from build123d import *

# Parameters (mm, degrees)
ESQUISSE1_W             = 120
ESQUISSE1_H             = 90
BOSS_EXTRU_1_DEPTH      = 2
ESQUISSE2_W             = 115
ESQUISSE2_H             = 85
ESQUISSE2_W_2           = 111
ESQUISSE2_H_2           = 82.04347826
BOSS_EXTRU_2_DEPTH      = 2
ENL_V_MAT_EXTRU_1_DEPTH = 2
CONG_1_R                = 3
CONG_2_R                = 0.5


with BuildPart() as part:
    # Esquisse1 → Boss.-Extru.1 (new body)
    with BuildSketch(Plane.XY):
        Rectangle(ESQUISSE1_W, ESQUISSE1_H)
    extrude(amount=BOSS_EXTRU_1_DEPTH)

    # Esquisse2 → Boss.-Extru.2 (add)
    with BuildSketch(Plane.XY.offset(2)):
        Rectangle(ESQUISSE2_W, ESQUISSE2_H)
        Rectangle(ESQUISSE2_W_2, ESQUISSE2_H_2, mode=Mode.SUBTRACT)
    extrude(amount=BOSS_EXTRU_2_DEPTH)

    # Esquisse3 → Enlèv. mat.-Extru.1 (cut)
    with BuildSketch(Plane(origin=(0, 0, 0), x_dir=(-1, 0, 0), z_dir=(0, 0, -1))):
        with BuildLine():
            Line((5.548380707, 39.874958244), (25.548380707, 39.874958244))
            ThreePointArc((25.548380707, 39.874958244), (30.548380707, 34.874958244), (25.548380707, 29.874958244))
            Line((25.548380707, 29.874958244), (5.548380707, 29.874958244))
            ThreePointArc((5.548380707, 29.874958244), (0.548380707, 34.874958244), (5.548380707, 39.874958244))
        make_face()
    extrude(amount=-ENL_V_MAT_EXTRU_1_DEPTH, mode=Mode.SUBTRACT)

    # Congé1
    cong_1_edges = [part.edges().sort_by_distance(p)[0] for p in [
        (-60, 45, 1),
        (60, 45, 1),
        (60, -45, 1),
        (-60, -45, 1),
    ]]
    fillet(cong_1_edges, radius=CONG_1_R)

    # Congé2
    cong_2_edges = [part.edges().sort_by_distance(p)[0] for p in [
        (-57.5, 42.5, 3),
        (-57.5, -42.5, 3),
        (57.5, -42.5, 3),
        (57.5, 42.5, 3),
    ]]
    fillet(cong_2_edges, radius=CONG_2_R)


solid = part.part
Work out the finished part from the listing and answer in its coordinate system (mm). A direction names the side the tool comes from. Give positions to 0.01 mm unless a question says otherwise; leave off trailing zeros. Loops run counter-clockwise (first coordinate to the right, second up) from the corner with the lowest first, then second, coordinate; pieces in that order, holes last. Notation, with made-up numbers: (62.5, 4) -> (109.5, 4) arc R17 ccw to (109.5, 22) -> close; hole circle Ø3 at (-35.75, -12). An arc over 180 degrees is marked (long way). Use a Markdown table: item, result. Add a question column.
1) The part is cut by section A-A, the plane x = -16. Determine the outline of the cut face in (y, z), plus the area to 3 significant figures.
2) Consider line 1 along Y through (x, z) = (51.5, 2.5); line 2 along X through (y, z) = (8.5, 3.1); line 3 along Y through (x, z) = (-25.5, 1.15). Determine where each line is inside the solid, lowest interval first.
3) The part is cut by section D-D, the plane y = 28. Determine the outline of the cut face in (x, z).
4) Which of the six approach directions +Z, -Z, +X, -X, +Y, -Y give full straight-line access (tool end or side, diameter ignored) to faces 1 (the cylindrical face through (59.1, -44.14, 1.01)), 2 (the cylindrical face through (-30.547, 34.985, 0.986))?
5) For a pull along Y with two mould halves and no side action, classify faces 3 (the flat face through (-1, 1, 2)), 4 (the flat face through (-1, 1, 0)), 5 (the cylindrical face through (-59.14, -44.1, 1.01)) as +Y half, -Y half, draft (parallel to the pull), parting line (faces both ways), or undercut.
6) The part is cut by section B-B, the plane z = 2.9. Determine the outline of the cut face in (x, y).
7) Each of these flat-tipped pins is pushed along its axis until it touches: P1, Ø1, axis at x = 11, z = 3, coming from the +Y side; P2, Ø24.5, axis at x = 20, y = 6.5, coming from the +Z side; P3, Ø0.6, axis at y = 18.5, z = 2.5, coming from the -X side; P4, Ø2, axis at x = 8.5, y = 31.5, coming from the -Z side. Where does it stop, or does it pass through?
8) The part is cut by section C-C, the plane x = 8.5. Determine the outline of the cut face in (y, z).
Reported:
| question | item | result |
|---|---|---|
| 1 | outline | (-45, 0) -> (29.87, 0) -> (29.87, 2) -> (-41.02, 2) -> (-41.02, 4) -> (-42.5, 4) -> (-42.5, 2) -> (-45, 2) -> close; (39.87, 0) -> (45, 0) -> (45, 2) -> (42.5, 2) -> (42.5, 4) -> (41.02, 4) -> (41.02, 2) -> (39.87, 2) -> close |
| 1 | area | 166 mm^2 |
| 2 | line 1 | y = -42.5 to -41.02, 41.02 to 42.5 |
| 2 | line 2 | x = -57.5 to -55.5, 55.5 to 57.5 |
| 2 | line 3 | y = -45 to 29.87, 39.87 to 45 |
| 3 | outline | (-60, 0) -> (60, 0) -> (60, 2) -> (57.5, 2) -> (57.5, 4) -> (55.5, 4) -> (55.5, 2) -> (-55.5, 2) -> (-55.5, 4) -> (-57.5, 4) -> (-57.5, 2) -> (-60, 2) -> close |
| 4 | face 1 | +Z, -Z, +X, -Y |
| 4 | face 2 | +Z, -Z |
| 5 | face 3 | undercut |
| 5 | face 4 | draft |
| 5 | face 5 | -Y half |
| 6 | outline | (-57.5, -42) arc R0.5 ccw to (-57, -42.5) -> (57, -42.5) arc R0.5 ccw to (57.5, -42) -> (57.5, 42) arc R0.5 ccw to (57, 42.5) -> (-57, 42.5) arc R0.5 ccw to (-57.5, 42) -> close; hole (-55.5, -41.02) -> (55.5, -41.02) -> (55.5, 41.02) -> (-55.5, 41.02) -> close |
| 7 | P1 | stops at y = 42.5 |
| 7 | P2 | stops at z = 2 |
| 7 | P3 | stops at x = -57.5 |
| 7 | P4 | stops at z = 0 |
| 8 | outline | (-45, 0) -> (45, 0) -> (45, 2) -> (42.5, 2) -> (42.5, 4) -> (41.02, 4) -> (41.02, 2) -> (-41.02, 2) -> (-41.02, 4) -> (-42.5, 4) -> (-42.5, 2) -> (-45, 2) -> close |
